from build123d import *

# Parameters (mm, degrees)
SKETCH_1_R          = 15
SKETCH_1_W          = 10.2
SKETCH_1_H          = 10.2
EXTRUDE_1_DEPTH     = 80
SKETCH1_R           = 19
SKETCH1_W           = 10.2
SKETCH1_H           = 10.2
BOSS_EXTRUDE1_DEPTH = 3
CHAMFER1_SIZE       = 1
CHAMFER1_SIZE2      = 2.747477419


with BuildPart() as part:
    # Эскиз1 → Бобышка-Вытянуть1 (new body)
    with BuildSketch(Plane(origin=(0, 0, 0), x_dir=(1, 0, 0), z_dir=(0, 1, 0))):
        Circle(SKETCH_1_R)
        Rectangle(SKETCH_1_W, SKETCH_1_H, mode=Mode.SUBTRACT)
    extrude(amount=EXTRUDE_1_DEPTH)

    # Sketch1 → Boss-Extrude1 (add)
    with BuildSketch(Plane(origin=(0, 80, 0), x_dir=(1, 0, 0), z_dir=(0, 1, 0))):
        Circle(SKETCH1_R)
        Rectangle(SKETCH1_W, SKETCH1_H, mode=Mode.SUBTRACT)
    extrude(amount=-BOSS_EXTRUDE1_DEPTH)

    # Chamfer1
    chamfer1_edges = [part.edges().sort_by_distance(p)[0] for p in [
        (0, 80, -5.1),
        (-5.1, 80, 0),
        (0, 80, 5.1),
        (5.1, 80, 0),
    ]]
    chamfer1_side = [part.faces().sort_by_distance(p)[0] for p in [
        (-18.462598846, 80, 0),
    ]]
    chamfer(chamfer1_edges, length=CHAMFER1_SIZE, length2=CHAMFER1_SIZE2, reference=chamfer1_side[0])


solid = part.part
Work out the finished part from the listing and answer in its coordinate system (mm). A direction names the side the tool comes from. Give positions to 0.01 mm unless a question says otherwise; leave off trailing zeros. Write each loop counter-clockwise with the first axis right and the second up, starting at its lowest first coordinate (ties: lowest second). Pieces come first, ordered by that corner, then holes. Notation, with made-up numbers: M -17,65.5 L 34,65.5 A22 ccw 34,83.5 Z; hole C 84,44.5 d4. An arc over 180 degrees is marked long. Answer as CSV lines item,"result".
Q1. Find the intervals of material crossed by probe 1 along Y at (x, z) = (-1.5, 15); probe 2 along Z at (x, y) = (-2, 50.5); probe 3 along X at (y, z) = (71, 2.5), in increasing order. Write a range as [from, to].
A:
probe 1,"y = [77, 80]"
probe 2,"z = [-14.87, -5.1], [5.1, 14.87]"
probe 3,"x = [-14.79, -5.1], [5.1, 14.79]"
Q2. The mould has two halves that part along Z. Classify faces 5 (the cylindrical face through (-14.985, 37.961, -0.66)), 6 (the flat face through (5.1, 38, 0)), 7 (the flat face through (6, 0, 0)): +Z half, -Z half, draft (parallel to the pull), parting line (faces both ways), or undercut.
A:
face 5,"parting line"
face 6,"undercut"
face 7,"draft"
Q3. A cutting plane is placed at A-A on z = 0. Write down the section's boundary in (x, y).
A:
outline,"M -19,77 L -15,77 L -15,0 L -5.1,0 L -5.1,77.25 L -6.1,80 L -19,80 Z; M 5.1,0 L 15,0 L 15,77 L 19,77 L 19,80 L 6.1,80 L 5.1,77.25 Z"
Q4. A tool of negligible diameter and unlimited length cuts with its end or side. For faces 1 (the flat face through (-0.085, 78.607, -5.593)), 2 (the flat face through (8, 80, 0)), 3 (the flat face through (14, 77, -6)), 4 (the flat face through (0, 38, 5.1)), from which of +Z, -Z, +X, -X, +Y, -Y can it reach the whole face along a straight path? Write none if from no direction.
A:
face 1,"+Y"
face 2,"+Z, -Z, +X, -X, +Y"
face 3,"-Y"
face 4,"+Y, -Y"
Q5. A cutting plane is placed at D-D on x = -8. Write down the section's boundary in (y, z).
A:
outline,"M 0,-12.69 L 77,-12.69 L 77,-17.23 L 80,-17.23 L 80,17.23 L 77,17.23 L 77,12.69 L 0,12.69 Z"
Q6. A cutting plane is placed at C-C on y = 18. Write down the section's boundary in (x, z), plus the area to 3 significant figures.
A:
outline,"C 0,0 d30; hole M -5.1,-5.1 L 5.1,-5.1 L 5.1,5.1 L -5.1,5.1 Z"
area,"603 mm²"
Q7. Given P1, Ø4, axis at y = 46, z = -0.5, coming from the -X side; P2, Ø5, axis at x = -0.5, y = 56, coming from the +Z side; P3, Ø1, axis at y = 69, z = 6, coming from the +X side, each flat-ended and moving along its own axis, determine where each tip first touches the part or whether it passes through.
A:
P1,"stops at x = -15"
P2,"stops at z = 15"
P3,"stops at x = 13.96"
Q8. A cutting plane is placed at B-B on x = 0. Write down the section's boundary in (y, z).
A:
outline,"M 0,-15 L 77,-15 L 77,-19 L 80,-19 L 80,-6.1 L 77.25,-5.1 L 0,-5.1 Z; M 0,5.1 L 77.25,5.1 L 80,6.1 L 80,19 L 77,19 L 77,15 L 0,15 Z"
